Autodesk Inventor part; units mm, degrees
ref_plane "YZ Plane" through (0, 0, 0) normal (1, 0, 0) x (0, 1, 0)
ref_plane "XZ Plane" through (0, 0, 0) normal (0, 1, 0) x (-1, 0, 0)
ref_plane "XY Plane" through (0, 0, 0) normal (0, 0, 1) x (1, 0, 0)
sketch "Sketch1" plane through (0, 0, 0) normal (0, 1, 0) x (-1, 0, 0)
  line L0 (0, 0) -> (0, 50)
  line L1 (0, 50) -> (-25, 50)
  line L2 (-25, 50) -> (-25, 0)
  line L3 (-25, 0) -> (0, 0)
  circle A0 centre (-12.5, 25) radius 6.35
  dimension "d0" = 50
  dimension "d1" = 25
  dimension "d2" = 12.7
extrude "Extrusion1" add sketch "Sketch1" against normal blind 6
sketch "Sketch2" plane through (0, -6, 0) normal (0, -1, 0) x (1, 0, 0)
  line L0 (0, 50) -> (0, 0)
  line L1 (0, 50) -> (6, 50)
  line L2 (25, 50) -> (0, 50)
  line L3 (6, 50) -> (6, 0)
  line L4 (0, 0) -> (25, 0)
  line L5 (6, 0) -> (0, 0)
  line L6 (0, 0) -> (0, 50)
  dimension "d5" = 6
extrude "Extrusion2" add sketch "Sketch2" along normal blind 19
sketch "Sketch3" plane through (6, -6, 50) normal (1, 0, 0) x (0, 0, -1)
  circle A0 centre (16.6667, -6.5) radius 3.25
  circle A1 centre (33.3333, -6.5) radius 3.25
  point P0 (50, 6)
  dimension "d8" = 6.5
  dimension "d9" = 6.5
hole "Hole1" at (6, -12.5, 33.3333) at (6, -12.5, 16.6667) direction (-1, 0, 0) diameter 6.5 depth 111
properties part number "Roter_shaft_support_top"
Can you work these out from the model? Positions are in its coordinate system, mm. A direction names the side the tool comes from. Coordinates: 2 decimals unless noted, no trailing zeros. Loops run counter-clockwise (first coordinate to the right, second up) from the corner with the lowest first, then second, coordinate; pieces in that order, holes last. Notation, with made-up numbers: (42, 17.5) -> (66, 17.5) arc R22 cw to (66, 25.5) -> close; hole circle Ø4 at (-25, -37.5). An arc over 180 degrees is marked (long way). Put each result on its own line as item: value. Start each with the question number.
Q1. For faces 1 (the face through (7, -4, 50)), 2 (the face through (20, -6, 25)), which set-ups out of +Z, -Z, +X, -X, +Y, -Y let a thin tool reach every point of the face, with its end or its side?
Q2. I want a section at C-C (y = -12.5). Write out the boundary of the cut face in (x, z).
Q3. I want a section at D-D (y = -2.5). Write out the boundary of the cut face in (x, z).
Q4. I want a section at B-B (z = 25). Write out the boundary of the cut face in (x, y), plus the area to 3 significant figures.
Q5. Thinking about a two-plate mould opening in Z: for faces 3 (the face through (4, -7, 0)), 4 (the face through (2.958, -13.476, 30.233)), 5 (the face through (6, -15, 25)), which applies, pulls with the +Z half, pulls with the -Z half, needs draft (parallel to the pull), parting line crosses it, or undercut?
Q6. If I drill on line 1 (Z direction, x = 4.5, y = -12.5); line 2 (Z direction, x = 2.5, y = -10); line 3 (Z direction, x = 12.5, y = -3.6), over which ranges is the centre line in solid material (lowest first)? Write a range as [from, to].
Q7. I'm going to push flat-ended pins straight in: P1, Ø8, axis at x = 12.5, y = -12.5, coming from the +Z side; P2, Ø5.5, axis at y = -20, z = 28.5, coming from the +X side. Where does each tip first touch, or does it pass through?
Q8. I want a section at A-A (x = 12.5). Write out the boundary of the cut face in (y, z), plus the area to 3 significant figures.
Taken from the geometry:
1. face 1: +Z, +X, -X, +Y, -Y
1. face 2: +Z, -Z, +X, -Y
2. outline: (0, 0) -> (6, 0) -> (6, 13.42) -> (0, 13.42) -> close; (0, 19.92) -> (6, 19.92) -> (6, 30.08) -> (0, 30.08) -> close; (0, 36.58) -> (6, 36.58) -> (6, 50) -> (0, 50) -> close
3. outline: (0, 0) -> (25, 0) -> (25, 50) -> (0, 50) -> close; hole circle Ø12.7 at (12.5, 25)
4. outline: (0, -25) -> (6, -25) -> (6, -6) -> (6.15, -6) -> (6.15, 0) -> (0, 0) -> close; (18.85, -6) -> (25, -6) -> (25, 0) -> (18.85, 0) -> close
4. area: 188 mm2
5. face 3: pulls with the -Z half
5. face 4: undercut
5. face 5: needs draft
6. line 1: z = [0, 13.42], [19.92, 30.08], [36.58, 50]
6. line 2: z = [0, 14.59], [18.74, 31.26], [35.41, 50]
6. line 3: z = [0, 18.65], [31.35, 50]
7. P1: passes through
7. P2: stops at x = 6
8. outline: (-6, 0) -> (0, 0) -> (0, 18.65) -> (-6, 18.65) -> close; (-6, 31.35) -> (0, 31.35) -> (0, 50) -> (-6, 50) -> close
8. area: 224 mm2
